Verification items for the finished model (mm, model axes). Face numbers are marked on the shaded views. Round coordinates to 2 decimals unless told otherwise and drop trailing zeros. Order: outer loops, then holes, each group sorted by start corner. A loop starts at its lowest first (then second) coordinate and runs counter-clockwise, first axis right, second up. Notation, with made-up numbers: (4.25, -15) -> (59.25, -15) arc R20 ccw to (59.25, 12) -> close; hole circle Ø5 at (61.5, 32). An arc over 180 degrees is marked (long way). Put each result on its own line as item: value.
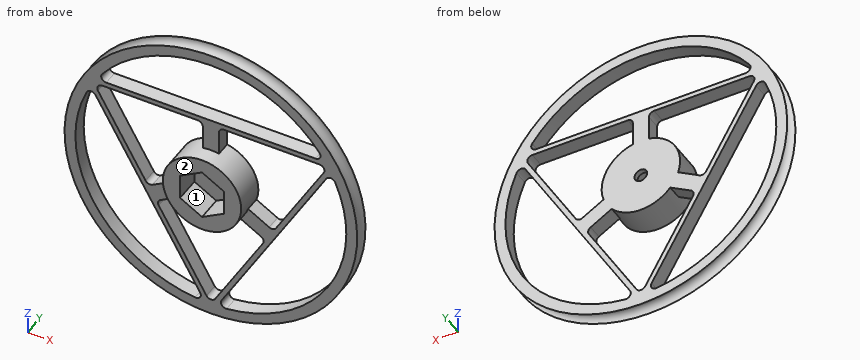
from build123d import *

# Parameters (mm, degrees)
SKETCH1_R           = 36.785134715
BOSS_EXTRUDE1_DEPTH = 3.683
SKETCH2_R           = 1.8415
BOSS_EXTRUDE2_START = -7.62
SKETCH5_R           = 9.858095427
BOSS_EXTRUDE2_DEPTH = 7.62
SKETCH6_R           = 1.5875
CUT_EXTRUDE1_DEPTH  = 53.577149714
CUT_EXTRUDE3_DEPTH  = 6.35


with BuildPart() as part:
    # Sketch1 → Boss-Extrude1 (new body)
    with BuildSketch(Plane(origin=(0, 0, 0), x_dir=(1, 0, 0), z_dir=(0, 1, 0))):
        with Locations(Location((0, 0, 0), (0, 0, 270))):
            Circle(SKETCH1_R)
        with BuildLine():
            Line((-1.099852263, 32.146289174), (-13.115875302, 11.333926765))
            ThreePointArc((-13.115875302, 11.333926765), (-13.242748838, 10.370226578), (-12.651023039, 9.599074503))
            Line((-12.651023039, 9.599074503), (-7.368281269, 6.549082119))
            ThreePointArc((-7.368281269, 6.549082119), (-8.559992893, 4.889638753), (-9.384056343, 3.020187413))
            Line((-9.384056343, 3.020187413), (-14.683023039, 6.079547262))
            ThreePointArc((-14.683023039, 6.079547262), (-15.646723226, 6.206420798), (-16.417875302, 5.614694999))
            Line((-16.417875302, 5.614694999), (-28.389429193, -15.120644587))
            ThreePointArc((-28.389429193, -15.120644587), (-28.389429193, -16.390644587), (-27.289576931, -17.025644587))
            Line((-27.289576931, -17.025644587), (-3.302, -17.025644587))
            ThreePointArc((-3.302, -17.025644587), (-2.403974388, -16.653670199), (-2.032, -15.755644587))
            Line((-2.032, -15.755644587), (-2.032, -9.646399404))
            ThreePointArc((-2.032, -9.646399404), (0, -9.858095427), (2.032, -9.646399404))
            Line((2.032, -9.646399404), (2.032, -15.755644587))
            ThreePointArc((2.032, -15.755644587), (2.403974388, -16.653670199), (3.302, -17.025644587))
            Line((3.302, -17.025644587), (27.289576931, -17.025644587))
            ThreePointArc((27.289576931, -17.025644587), (28.389429193, -16.390644587), (28.389429193, -15.120644587))
            Line((28.389429193, -15.120644587), (16.395640728, 5.65320641))
            ThreePointArc((16.395640728, 5.65320641), (15.624488653, 6.24493221), (14.660788465, 6.118058673))
            Line((14.660788465, 6.118058673), (9.370026939, 3.063436081))
            ThreePointArc((9.370026939, 3.063436081), (8.537361073, 4.929047714), (7.338026939, 6.582963322))
            Line((7.338026939, 6.582963322), (12.628788465, 9.637585914))
            ThreePointArc((12.628788465, 9.637585914), (13.220514265, 10.408737989), (13.093640728, 11.372438177))
            Line((13.093640728, 11.372438177), (1.099852263, 32.146289174))
            ThreePointArc((1.099852263, 32.146289174), (0, 32.781289174), (-1.099852263, 32.146289174))
        make_face(mode=Mode.SUBTRACT)
        with BuildLine():
            Line((-2.693461931, 31.926076262), (-28.995524051, -13.630431675))
            ThreePointArc((-28.995524051, -13.630431675), (-30.168979582, -14.26329703), (-31.261319719, -13.498895652))
            ThreePointArc((-31.261319719, -13.498895652), (-29.489281456, 17.025644587), (-3.940273302, 33.822544859))
            ThreePointArc((-3.940273302, 33.822544859), (-2.732112221, 33.258751239), (-2.693461931, 31.926076262))
        make_face(mode=Mode.SUBTRACT)
        with BuildLine():
            Line((2.693461931, 31.926076262), (28.995524051, -13.630431675))
            ThreePointArc((28.995524051, -13.630431675), (30.168979582, -14.26329703), (31.261319719, -13.498895652))
            ThreePointArc((31.261319719, -13.498895652), (29.489281456, 17.025644587), (3.940273302, 33.822544859))
            ThreePointArc((3.940273302, 33.822544859), (2.732112221, 33.258751239), (2.693461931, 31.926076262))
        make_face(mode=Mode.SUBTRACT)
        with BuildLine():
            Line((-26.302062121, -18.295644587), (26.302062121, -18.295644587))
            ThreePointArc((26.302062121, -18.295644587), (27.436867361, -18.995454209), (27.321046417, -20.323649206))
            ThreePointArc((27.321046417, -20.323649206), (0, -34.051289174), (-27.321046417, -20.323649206))
            ThreePointArc((-27.321046417, -20.323649206), (-27.436867361, -18.995454209), (-26.302062121, -18.295644587))
        make_face(mode=Mode.SUBTRACT)
    extrude(amount=BOSS_EXTRUDE1_DEPTH)

    # Sketch2 → Cut-Revolve2 (revolve, cut)
    with BuildSketch(Plane.XY, mode=Mode.PRIVATE) as cut_revolve2_sk:
        with Locations((36.785134715, 1.8415)):
            Circle(SKETCH2_R)
    revolve(cut_revolve2_sk.sketch.rotate(Axis((0, 0, 0), (0, 1, 0)), 90), axis=Axis((0, 0, 0), (0, 1, 0)), mode=Mode.SUBTRACT)

    # Sketch5 → Boss-Extrude2 (add)
    with BuildSketch(Plane(origin=(0, 3.683, 0), x_dir=(1, 0, 0), z_dir=(0, 1, 0)).offset(BOSS_EXTRUDE2_START)):
        with Locations(Location((0, 0, 0), (0, 0, 270))):
            Circle(SKETCH5_R)
    extrude(amount=BOSS_EXTRUDE2_DEPTH)

    # Sketch6 → Cut-Extrude1 (cut, through all)
    with BuildSketch(Plane.XZ.offset(3.937)):
        with Locations(Location((0, 0, 0), (0, 0, 270))):
            Circle(SKETCH6_R)
    extrude(amount=-CUT_EXTRUDE1_DEPTH, mode=Mode.SUBTRACT)

    # Sketch8 → Cut-Extrude3 (cut)
    with BuildSketch(Plane.XZ.offset(3.937)):
        Polygon((0, 6.35), (-5.499261314, 3.175), (-5.499261314, -3.175), (0, -6.35), (5.499261314, -3.175), (5.499261314, 3.175), align=None)
    extrude(amount=-CUT_EXTRUDE3_DEPTH, mode=Mode.SUBTRACT)


solid = part.part
Item 1: Release check for a two-part mould opening along Z. For the marked faces 1 and 2 record: +Z half, -Z half, draft (parallel to the pull), parting line (faces both ways), or undercut.
Check sheet entries:
face 1: undercut
face 2: draft
Item 2: Gauge pin test, flat ends, axial feed: pin 1 Ø6 at (x, z) = (-5, 14.5) entering from -Y; pin 2 Ø1.8 at (x, y) = (8.5, 1.5) entering from +Z; pin 3 Ø1.8 at (y, z) = (2, 12.5) entering from -X. Record the tip position at first contact, or that the pin passes through.
Check sheet entries:
pin 1: stops at y = 0
pin 2: stops at z = 34.42
pin 3: stops at x = -33.07
Item 3: Section check A-A on y = -1.75. Record the boundary of the cut face in (x, z) (3 decimals).
Check sheet entries:
outline: circle Ø19.716 at (0, 0); hole (-5.499, -3.175) -> (0, -6.35) -> (5.499, -3.175) -> (5.499, 3.175) -> (0, 6.35) -> (-5.499, 3.175) -> close
Item 4: Material ranges on L1, parallel to X at y = 0.5, z = -15; L2, parallel to Z at x = 7, y = 2.75; L3, parallel to X at y = 2.5, z = -13, recorded low to high. Write a range as [from, to].
Check sheet entries:
L1: x = [-32.2, -30.57], [-12.47, -11], [11, 12.47], [30.57, 32.2]
L2: z = [-34.48, -33.32], [-24.47, -21.93], [-6.94, 6.94], [17.03, 18.3], [33.32, 34.48]
L3: x = [-32.57, -31.47], [-13.62, -12.15], [12.15, 13.62], [31.47, 32.57]
Item 5: Section check B-B on z = 0. Record the boundary of the cut face in (x, y).
Check sheet entries:
outline: (-36.79, 0) -> (-34.05, 0) -> (-34.05, 3.68) -> (-36.79, 3.68) arc R1.84 cw to start; (-21.13, 0) -> (-19.66, 0) -> (-19.66, 3.68) -> (-21.13, 3.68) -> close; (-9.86, -3.94) -> (-5.5, -3.94) -> (-5.5, 2.41) -> (-1.59, 2.41) -> (-1.59, 3.68) -> (-9.86, 3.68) -> close; (1.59, 2.41) -> (5.5, 2.41) -> (5.5, -3.94) -> (9.86, -3.94) -> (9.86, 3.68) -> (1.59, 3.68) -> close; (19.66, 0) -> (21.13, 0) -> (21.13, 3.68) -> (19.66, 3.68) -> close; (34.05, 0) -> (36.79, 0) arc R1.84 cw to (36.79, 3.68) -> (34.05, 3.68) -> close
Item 6: Section check C-C on x = -19.5. State how many separate pieces and enclosed holes the cut face has, then the cut area to 3 significant figures.
Check sheet entries:
separate pieces: 4
enclosed holes: 0
area: 25.5 mm^2
